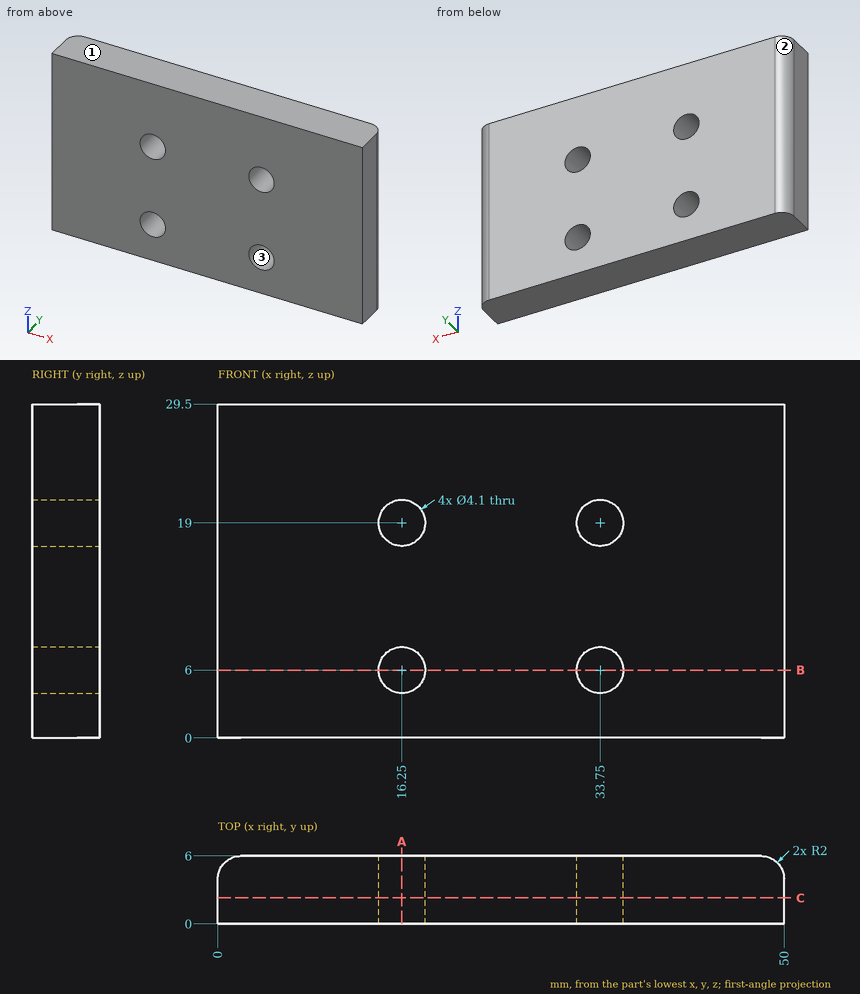
Geometry: see drawing. Coordinates: mm, zero at the bounding-box minimum. Coordinates: 2 decimals unless noted, no trailing zeros. Loops run counter-clockwise (first coordinate to the right, second up) from the corner with the lowest first, then second, coordinate; pieces in that order, holes last.
Q1. Cut plane B-B (z = 6). Output: boundary loops of the cut face in (x, y).
Q2. Cut plane C-C (y = 2.3). Output: boundary loops of the cut face in (x, z), then the cut area to 3 significant figures.
Q3. Cut plane A-A (x = 16.25). Output: boundary loops of the cut face in (y, z).
Q4. Draft query along X for the marked faces 1, 2 and 3. Return one class per face: +X half, -X half, draft (parallel to the pull), parting line (faces both ways), or undercut.
Q5. Material intervals for line 1 (X direction, y = 1.6, z = 19); line 2 (X direction, y = 5.7, z = 5); line 3 (Z direction, x = 35, y = 5.6), sorted ascending.
Working result:
1. outline: (0, 0) - (14.2, 0) - (14.2, 6) - (2, 6) arc R2 ccw to (0, 4) - close; (18.3, 0) - (31.7, 0) - (31.7, 6) - (18.3, 6) - close; (35.8, 0) - (50, 0) - (50, 4) arc R2 ccw to (48, 6) - (35.8, 6) - close
2. outline: (0, 0) - (50, 0) - (50, 29.5) - (0, 29.5) - close; hole circle Ø4.1 at (16.25, 6); hole circle Ø4.1 at (16.25, 19); hole circle Ø4.1 at (33.75, 6); hole circle Ø4.1 at (33.75, 19)
2. area: 1,420 mm2
3. outline: (0, 0) - (6, 0) - (6, 3.95) - (0, 3.95) - close; (0, 8.05) - (6, 8.05) - (6, 16.95) - (0, 16.95) - close; (0, 21.05) - (6, 21.05) - (6, 29.5) - (0, 29.5) - close
4. face 1: draft
4. face 2: -X half
4. face 3: undercut
5. line 1: x = 0 to 14.2, 18.3 to 31.7, 35.8 to 50
5. line 2: x = 0.95 to 14.46, 18.04 to 31.96, 35.54 to 49.05
5. line 3: z = 0 to 4.38, 7.62 to 17.38, 20.62 to 29.5
